```python
from build123d import *

# Parameters (mm, degrees)
SKETCH1_W                = 95
SKETCH1_H                = 33
BOSS_EXTRUDE1_DEPTH      = 12
SKETCH2_R                = 6
CUT_EXTRUDE1_DEPTH       = 12
SKETCH3_W                = 25
SKETCH3_H                = 68
BOSS_EXTRUDE2_DEPTH      = 28
BOSS_EXTRUDE2_DEPTH_BACK = 12
SKETCH4_R                = 20
BOSS_EXTRUDE3_DEPTH      = 25
SKETCH5_R                = 12.5
CUT_EXTRUDE2_DEPTH       = 25
SKETCH6_W                = 95
SKETCH6_H                = 55
BOSS_EXTRUDE4_DEPTH      = 12
SKETCH7_W                = 37
SKETCH7_H                = 20
CUT_EXTRUDE3_DEPTH       = 12
FILLET1_R                = 8


with BuildPart() as part:
    # Sketch1 → Boss-Extrude1 (new body)
    with BuildSketch(Plane.XY):
        with Locations((9.985654596, -9.139131357)):
            Rectangle(SKETCH1_W, SKETCH1_H)
    extrude(amount=-BOSS_EXTRUDE1_DEPTH)

    # Sketch2 → Cut-Extrude1 (cut)
    with BuildSketch(Plane.XY):
        with Locations((-25.014345404, -12.639131357)):
            Circle(SKETCH2_R)
        with Locations((16.485654596, -12.639131357)):
            Circle(SKETCH2_R)
    extrude(amount=-CUT_EXTRUDE1_DEPTH, mode=Mode.SUBTRACT)

    # Sketch3 → Boss-Extrude2 (add, two sides)
    with BuildSketch(Plane.XY) as boss_extrude2_sk:
        with Locations((44.985654596, 8.360868643)):
            Rectangle(SKETCH3_W, SKETCH3_H)
    extrude(amount=BOSS_EXTRUDE2_DEPTH)
    extrude(boss_extrude2_sk.sketch, amount=-BOSS_EXTRUDE2_DEPTH_BACK)

    # Sketch4 → Boss-Extrude3 (add)
    with BuildSketch(Plane(origin=(57.485654596, 0, 0), x_dir=(0, 0, -1), z_dir=(1, 0, 0))):
        with Locations((-8, 42.360868643)):
            Circle(SKETCH4_R)
    extrude(amount=-BOSS_EXTRUDE3_DEPTH)

    # Sketch5 → Cut-Extrude2 (cut)
    with BuildSketch(Plane(origin=(57.485654596, 0, 0), x_dir=(0, 0, -1), z_dir=(1, 0, 0))):
        with Locations((-8, 42.360868643)):
            Circle(SKETCH5_R)
    extrude(amount=-CUT_EXTRUDE2_DEPTH, mode=Mode.SUBTRACT)

    # Sketch6 → Boss-Extrude4 (add)
    with BuildSketch(Plane.XZ.offset(25.639131357)):
        with Locations((9.985654596, 15.5)):
            Rectangle(SKETCH6_W, SKETCH6_H)
    extrude(amount=BOSS_EXTRUDE4_DEPTH)

    # Sketch7 → Cut-Extrude3 (cut)
    with BuildSketch(Plane(origin=(0, -25.639131357, 0), x_dir=(1, 0, 0), z_dir=(0, 1, 0))):
        with Locations((0.985654596, -13)):
            Rectangle(SKETCH7_W, SKETCH7_H)
    extrude(amount=-CUT_EXTRUDE3_DEPTH, mode=Mode.SUBTRACT)

    # Fillet1
    fillet1_edges = [part.edges().sort_by_distance(p)[0] for p in [
        (32.485654596, 7.360868643, -6),
    ]]
    fillet(fillet1_edges, radius=FILLET1_R)


solid = part.part
```
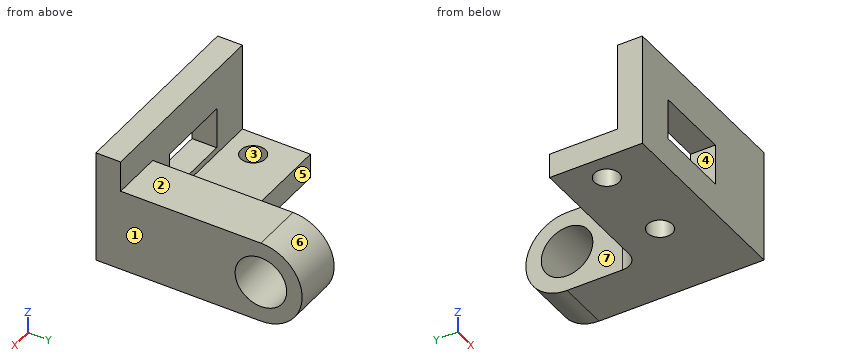
Work out the finished part from the listing and answer in its coordinate system (mm). Face numbers are marked on the shaded views. A direction names the side the tool comes from. Give positions to 0.01 mm unless a question says otherwise; leave off trailing zeros. Order: outer loops, then holes, each group sorted by start corner. A loop starts at its lowest first (then second) coordinate and runs counter-clockwise, first axis right, second up. Notation, with made-up numbers: (23, -26.5) - (49, -26.5) arc R29 ccw to (49, 7.5) - close; hole circle Ø10 at (-35, 1). An arc over 180 degrees is marked (long way). One line per item, written item: value. Start each with the question number.
1. Section D-D, the plane y = 19 is taken. Write down the section's boundary in (x, z), then the cut area to 3 significant figures.
2. Which of the six approach directions +Z, -Z, +X, -X, +Y, -Y give full straight-line access (tool end or side, diameter ignored) to the marked faces 4, 5, 6 and 7?
3. Consider line 1 (Y direction, x = 44.25, z = 8); line 2 (Y direction, x = 24.5, z = 14); line 3 (X direction, y = 40, z = -9). Determine where each line is inside the solid, lowest interval first.
4. Each of these flat-tipped pins is pushed along its axis until it touches: pin 1 Ø4 at (y, z) = (4.5, 17) entering from -X; pin 2 Ø12.5 at (x, y) = (-1.5, -0.5) entering from +Z; pin 3 Ø4 at (x, z) = (35.5, -4) entering from +Y. Where does it stop, or does it pass through?
5. Section C-C, the plane x = -12 is taken. Write down the section's boundary in (y, z).
6. Section A-A, the plane x = 40.5 is taken. Write down the section's boundary in (y, z), then the cut area to 3 significant figures.
7. For a pull along X with two mould halves and no side action, classify the marked faces 1, 2 and 3 as released by +X, released by -X, zero draft, split by the parting line, or undercut.
8. Section B-B, the plane z = 8 is taken. Write down the section's boundary in (x, y).
Filled sheet:
1. outline: (32.49, -12) - (57.49, -12) - (57.49, 28) - (32.49, 28) - close
1. area: 1,000 mm²
2. face 4: +Y, -Y
2. face 5: +Z, -Z, -X, +Y
2. face 6: +X, -X, +Y
2. face 7: +Z, -X, +Y
3. line 1: -37.64 to 29.86, 54.86 to 62.36
3. line 2: -37.64 to -25.64
3. line 3: 32.49 to 57.49
4. pin 1: x = 32.49
4. pin 2: z = 0
4. pin 3: y = 59.68
5. outline: (-37.64, -12) - (7.36, -12) - (7.36, 0) - (-25.64, 0) - (-25.64, 3) - (-37.64, 3) - close; (-37.64, 23) - (-25.64, 23) - (-25.64, 43) - (-37.64, 43) - close
6. outline: (-37.64, -12) - (42.36, -12) arc R20 ccw to (42.36, 28) - (-25.64, 28) - (-25.64, 43) - (-37.64, 43) - close; hole circle Ø25 at (42.36, 8)
6. area: 3,520 mm²
7. face 1: released by +X
7. face 2: zero draft
7. face 3: undercut
8. outline: (-37.51, -37.64) - (-17.51, -37.64) - (-17.51, -25.64) - (-37.51, -25.64) - close; (19.49, -37.64) - (57.49, -37.64) - (57.49, 29.86) - (32.49, 29.86) - (32.49, -25.64) - (19.49, -25.64) - close; (32.49, 54.86) - (57.49, 54.86) - (57.49, 62.36) - (32.49, 62.36) - close
